Autodesk Inventor part; units mm, degrees
ref_plane "YZ Plane" through (0, 0, 0) normal (1, 0, 0) x (0, 1, 0)
ref_plane "XZ Plane" through (0, 0, 0) normal (0, 1, 0) x (-1, 0, 0)
ref_plane "XY Plane" through (0, 0, 0) normal (0, 0, 1) x (1, 0, 0)
sketch "Sketch1" plane through (0, 0, 0) normal (0, 1, 0) x (-1, 0, 0)
  line L0 (50, 130) -> (-50, 130)
  line L1 (-50, 130) -> (-50, -130)
  line L2 (-50, -130) -> (50, -130)
  line L3 (50, -130) -> (50, 130)
  line L4 (50, 130) -> (-50, -130) construction
  line L5 (-50, 130) -> (50, -130) construction
  line L6 (57.5, 137.5) -> (-57.5, 137.5)
  line L7 (-57.5, 137.5) -> (-57.5, -137.5)
  line L8 (-57.5, -137.5) -> (57.5, -137.5)
  line L9 (57.5, -137.5) -> (57.5, 137.5)
  line L10 (57.5, 137.5) -> (-57.5, -137.5) construction
  line L11 (-57.5, 137.5) -> (57.5, -137.5) construction
  circle A0 centre (50, 130) radius 2.5
  circle A1 centre (-50, 130) radius 2.5
  circle A2 centre (-50, -130) radius 2.5
  circle A3 centre (50, -130) radius 2.5
  point P0 (0, 0)
  dimension "d0" = 100
  dimension "d1" = 260
  dimension "d2" = 115
  dimension "d3" = 275
  dimension "d4" = 5
  dimension "d5" = 5
  dimension "d6" = 5
  dimension "d7" = 5
extrude "Extrusion1" add sketch "Sketch1" along normal blind 6 contours L0 A0 L3 A3 L2 A2 L1 A1 | L9 L8 L7 L6
sketch "Sketch2" plane through (0, 6, 0) normal (0, 1, 0) x (1, 0, 0)
  circle A0 centre (0, 0) radius 2.5
  line L0 (0, 0) -> (42, 0)
  line L1 (42, 0) -> (0, 0)
  line L2 (0, 0) -> (-28, 0)
  line L3 (-28, 0) -> (-28, 28)
  line L4 (-28, 28) -> (-28, -28)
  line L5 (42, 0) -> (42, 20)
  line L6 (42, 20) -> (42, -20)
  circle A1 centre (-28, -28) radius 1.25
  circle A2 centre (-28, 28) radius 1
  circle A3 centre (42, 20) radius 1.25
  circle A4 centre (42, -20) radius 1.25
  line L7 (-21.6952, -23.1643) -> (-21.6952, -28.1643)
  line L8 (-21.6952, -28.1643) -> (-21.6952, -23.1643)
  line L9 (-21.6952, -23.1643) -> (-21.6952, -18.1643)
  line L10 (-21.6952, -18.1643) -> (13.3048, -18.1643)
  line L11 (13.3048, -18.1643) -> (13.3048, -28.1643)
  line L12 (13.3048, -28.1643) -> (-21.6952, -28.1643)
  dimension "d10" = 5
  dimension "d11" = 42
  dimension "d12" = 42
  dimension "d13" = 28
  dimension "d14" = 28
  dimension "d15" = 56
  dimension "d16" = 20
  dimension "d17" = 40
  dimension "d18" = 2.5
  dimension "d19" = 2
  dimension "d20" = 2.5
  dimension "d21" = 2.5
  dimension "d22" = 5
  dimension "d23" = 5
  dimension "d24" = 5
  dimension "d25" = 35
extrude "Extrusion2" cut sketch "Sketch2" against normal blind 6
sketch "Sketch3" plane through (0, 6, 0) normal (0, 1, 0) x (1, 0, 0)
  point P0 (0, 0)
sketch "Sketch4" plane through (0, 6, 0) normal (0, 1, 0) x (1, 0, 0)
  line L0 (-57.5, 137.5) -> (-57.5, -137.5)
  line L1 (-57.5, -137.5) -> (-57.5, 0)
  line L2 (-21.6952, -18.1643) -> (-21.6952, -28.1643)
  line L3 (-21.6952, -28.1643) -> (-75.3295, -28.1643)
  line L4 (-75.3295, -28.1643) -> (-57.5, -28.1643)
  line L5 (-57.5, -137.5) -> (-57.5, -28.1643)
  line L6 (-57.5, -28.1643) -> (-57.5, -82.8322)
  line L7 (-57.5, -82.8322) -> (-27.1083, -82.8322)
  line L8 (-27.1083, -82.8322) -> (0, -82.8322)
  line L9 (0, -82.8322) -> (72.7953, -82.8322)
  line L10 (72.7953, -82.8322) -> (0, -82.8322)
  line L11 (0, -95.2871) -> (0, -82.8322)
  line L12 (0, -95.2871) -> (-27.1083, -95.2871)
  line L13 (-27.1083, -95.2871) -> (0, -95.2871)
  line L14 (33.9195, -95.2871) -> (0, -95.2871)
  circle A0 centre (-27.1083, -95.2871) radius 11.5
  circle A1 centre (33.9195, -95.2871) radius 6.5
  point P0 (0, 0)
  dimension "d28" = 23
  dimension "d29" = 13
extrude "Extrusion3" cut sketch "Sketch4" against normal blind 10
sketch "Sketch5" plane through (0, 6, 0) normal (0, 1, 0) x (1, 0, 0)
  line L0 (-57.5, -137.5) -> (57.5, -137.5)
  line L1 (-57.5, -137.5) -> (-64.1, -137.5)
  line L2 (57.5, 137.5) -> (-57.5, 137.5)
  line L3 (-57.5, 137.5) -> (-64.1, 137.5)
  line L4 (-64.1, 137.5) -> (-64.1, -137.5)
  line L5 (-64.1, 137.5) -> (-64.1, 145)
  line L6 (-64.1, 145) -> (57.5, 145)
  line L7 (57.5, 145) -> (57.5, 137.5)
  line L8 (57.5, 145) -> (62, 145)
  line L9 (62, 145) -> (62, -137.5)
  line L10 (57.5, -137.5) -> (57.5, 137.5)
  line L11 (62, -137.5) -> (57.5, -137.5)
  line L12 (-64.1, -137.5) -> (-64.1, -140.5)
  line L13 (-64.1, -140.5) -> (62, -140.5)
  line L14 (62, -140.5) -> (62, -137.5)
  line L15 (-57.5, -137.5) -> (-57.5, 137.5)
  line L16 (57.5, 137.5) -> (57.5, -137.5)
  point P0 (0, 0)
  dimension "d32" = 6.6
  dimension "d33" = 6.6
  dimension "d34" = 7.5
  dimension "d35" = 4.5
  dimension "d36" = 3
extrude "Extrusion4" add sketch "Sketch5" against normal blind 6 contours L0 L11 L14 L13 L12 L1 | L1 L4 L3 L15 | L10 L7 L8 L9 L11 | L3 L5 L6 L7 L2
properties part number "platform_plate" material "Acrylic"
Build history of the part. All positions in model axes, mm. A direction names the side the tool comes from. Coordinates: 2 decimals unless noted, no trailing zeros. Order: outer loops, then holes, each group sorted by start corner. A loop starts at its lowest first (then second) coordinate and runs counter-clockwise, first axis right, second up. Notation, with made-up numbers: (52.25, 34) -> (95.25, 34) arc R16 cw to (95.25, 64) -> close; hole circle Ø1 at (18.5, 3). An arc over 180 degrees is marked (long way). Answer in a Markdown table with one row per item. Add a question column.
Q1. Drop a flat-ended pin along its axis: pin 1 (1.5 mm diameter, centred on x = 42, z = 20, fed in from -Y). Give the stop position or say it passes through.
Q2. Band-saw the part on C-C, the plane x = -50. List the corners of the cut face in (y, z).
Q3. Mould opens along Z. For faces 1 (the face through (-2, 3, 140.5)), 2 (the face through (-2, 3, -145)), 3 (the face through (-0.54, 3.04, 2.44)), 4 (the face through (14, 0, 0)) say: +Z half, -Z half, draft (parallel to the pull), parting line (faces both ways), or undercut.
Q4. Which spindle directions (+Z, -Z, +X, -X, +Y, -Y) get a long thin tool onto all of the face, cutting with end or side? Do faces 5 (the face through (14, 6, 0)), 6 (the face through (-21.695, 3, 23)). Say none if no direction does.
Q5. Band-saw the part on D-D, the plane y = 4.9. Give the number of separate pieces and of enclosed holes in the cut face, then the cut area to 3 significant figures.
Q6. Wall check: line 1 along Z through (x, y) = (42, 3.8); line 2 along X through (y, z) = (1.9, 130); line 3 along X through (y, z) = (1.2, 28). Give the ranges that are in metal, low to high. Write a range as [from, to].
Q7. Band-saw the part on B-B, the plane x = 8. List the corners of the cut face in (y, z).
Q8. Band-saw the part on A-A, the plane z = 130. List the corners of the cut face in (x, y).
Answers follow:
| question | item | result |
|---|---|---|
| 1 | pin 1 | through |
| 2 | outline | (0, -145) -> (6, -145) -> (6, -132.5) -> (0, -132.5) -> close; (0, -127.5) -> (6, -127.5) -> (6, 127.5) -> (0, 127.5) -> close; (0, 132.5) -> (6, 132.5) -> (6, 140.5) -> (0, 140.5) -> close |
| 3 | face 1 | +Z half |
| 3 | face 2 | -Z half |
| 3 | face 3 | undercut |
| 3 | face 4 | draft |
| 4 | face 5 | +Z, -Z, +X, -X, +Y |
| 4 | face 6 | +Y, -Y |
| 5 | separate pieces | 1 |
| 5 | enclosed holes | 12 |
| 5 | area | 35,000 mm^2 |
| 6 | line 1 | [-145, -21.25], [-18.75, 18.75], [21.25, 140.5] |
| 6 | line 2 | [-64.1, -52.5], [-47.5, 47.5], [52.5, 62] |
| 6 | line 3 | [-64.1, -29.25], [-26.75, -21.7], [13.3, 62] |
| 7 | outline | (0, -145) -> (6, -145) -> (6, 18.16) -> (0, 18.16) -> close; (0, 28.16) -> (6, 28.16) -> (6, 140.5) -> (0, 140.5) -> close |
| 8 | outline | (-64.1, 0) -> (-52.5, 0) -> (-52.5, 6) -> (-64.1, 6) -> close; (-47.5, 0) -> (47.5, 0) -> (47.5, 6) -> (-47.5, 6) -> close; (52.5, 0) -> (62, 0) -> (62, 6) -> (52.5, 6) -> close |
